Here's how the part is built. I have some questions about the finished solid (model axes, mm). Face numbers are marked on the shaded views. Give positions to 0.01 mm unless a question says otherwise; leave off trailing zeros. Loops run counter-clockwise (first coordinate to the right, second up) from the corner with the lowest first, then second, coordinate; pieces in that order, holes last. Notation, with made-up numbers: M -13,53.5 L 39,53.5 A12 ccw 39,74.5 Z; hole C 63,37 d2. An arc over 180 degrees is marked long. Answer as CSV lines item,"result". Start each with the question number.
Item 1: If we mould it in two halves opening along X, with no side actions, what happens to the marked faces 1 and 2? For each: released by +X, released by -X, zero draft, split by the parting line, or undercut.
Item 2: Will these pins go through, and if not, where does the flat tip stop? P1, Ø1, axis at x = 17, y = -446, coming from the +Z side; P2, Ø5, axis at y = -41, z = 0.5, coming from the +X side; P3, Ø1.5, axis at x = 27.5, y = -28.5, coming from the -Z side; P4, Ø2.5, axis at y = 705, z = -0.5, coming from the -X side.
Item 3: If I drill on line 1 along Y through (x, z) = (36, 0.25); line 2 along Z through (x, y) = (-12, -644); line 3 along Z through (x, y) = (-15.5, 331.5), over which ranges is the centre line in solid material (lowest first)? Write a range as from..to.
Item 4: I want a section at B-B on x = 2.5. List the corners of the cut face in (y, z) for me, plus the area to 3 significant figures.
Item 5: I want a section at A-A on y = 554. List the corners of the cut face in (x, z) for me.
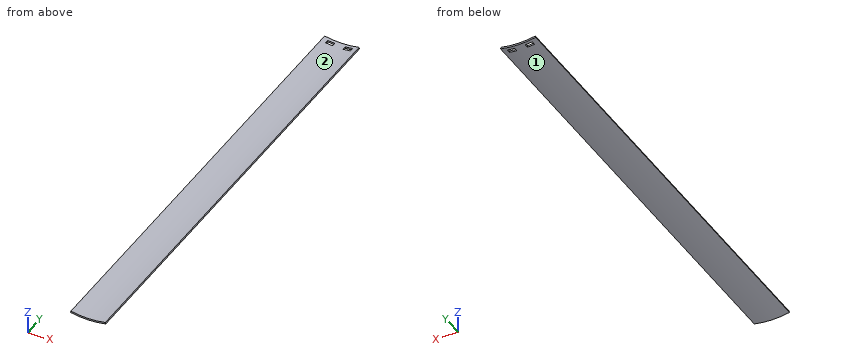
from build123d import *

# Parameters (mm, degrees)
BOSS_EXTRUDE1_DEPTH     = 720
CUT_EXTRUDE6_DEPTH      = 723.121476834
CUT_EXTRUDE6_DEPTH_BACK = 723.121476834
SKETCH8_W               = 22.5
SKETCH8_H               = 12.5


with BuildPart() as part:
    # Sketch3 → Boss-Extrude1 (new, symmetric)
    with BuildSketch(Plane(origin=(0, 0, 0), x_dir=(1, 0, 0), z_dir=(0, 1, 0))):
        with BuildLine():
            Line((-55, -0.016406212), (-53.942307692, -4.903254581))
            ThreePointArc((-53.942307692, -4.903254581), (0, 0.867478597), (53.942307692, -4.903254581))
            Line((53.942307692, -4.903254581), (55, -0.016406212))
            ThreePointArc((55, -0.016406212), (0, 5.867478597), (-55, -0.016406212))
        make_face()
    extrude(amount=BOSS_EXTRUDE1_DEPTH, both=True)

    # Sketch8 → Cut-Extrude6 (cut, two sides: drawn at the far end of the back side and taken through both)
    with BuildSketch(Plane.XY.offset(-CUT_EXTRUDE6_DEPTH_BACK)):
        with Locations((-27.692307692, 703.75)):
            Rectangle(SKETCH8_W, SKETCH8_H)
        with Locations((27.692307692, 703.75)):
            Rectangle(SKETCH8_W, SKETCH8_H)
    extrude(amount=CUT_EXTRUDE6_DEPTH + CUT_EXTRUDE6_DEPTH_BACK, mode=Mode.SUBTRACT)


solid = part.part
Result:
1,face 1,"split by the parting line"
1,face 2,"undercut"
2,P1,"z = -0.27"
2,P2,"x = 55"
2,P3,"z = -4.49"
2,P4,"x = -55"
3,line 1,"-720..697.5, 710..720"
3,line 2,"-5.59..-0.58"
3,line 3,"-5.41..-0.4"
4,outline,"M -720,-5.86 L 720,-5.86 L 720,-0.86 L -720,-0.86 Z"
4,area,"7,200 mm^2"
5,outline,"M -55,0.02 A260 ccw 55,0.02 L 53.94,4.9 A255 cw -53.94,4.9 Z"
